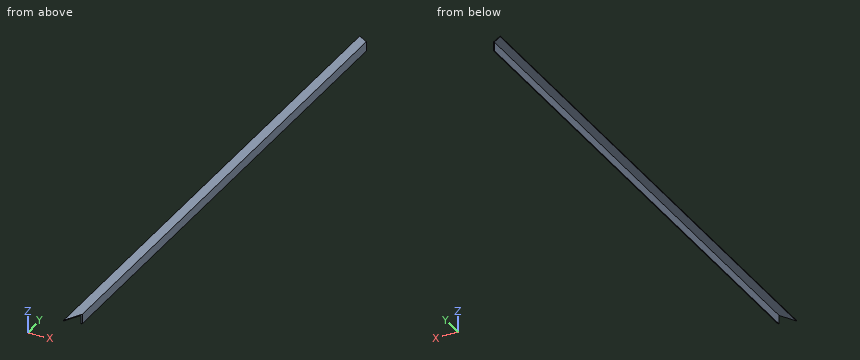
Autodesk Inventor part; units mm, degrees
ref_plane "YZ Plane" through (0, 0, 0) normal (1, 0, 0) x (0, 1, 0)
ref_plane "XZ Plane" through (0, 0, 0) normal (0, 1, 0) x (-1, 0, 0)
ref_plane "XY Plane" through (0, 0, 0) normal (0, 0, 1) x (1, 0, 0)
sketch "Sketch1" plane through (0, 0, 0) normal (0, 1, 0) x (-1, 0, 0)
  line L0 (0, 0) -> (38.1, 0)
  line L1 (38.1, 0) -> (38.1, -3.175)
  line L2 (38.1, -3.175) -> (3.175, -3.175)
  line L3 (3.175, -3.175) -> (3.175, -38.1)
  line L4 (3.175, -38.1) -> (0, -38.1)
  line L5 (0, -38.1) -> (0, 0)
  dimension "d0" = 3.175
  dimension "d1" = 3.175
  dimension "d2" = 38.1
  dimension "d3" = 38.1
extrude "Extrusion1" add sketch "Sketch1" along normal blind 2133.6
sketch "Sketch2" plane through (0, 0, 0) normal (0, 0, 1) x (1, 0, 0)
  line L0 (0, 0) -> (-38.1, 0)
  line L1 (-38.1, 0) -> (0, 0)
  line L2 (0, 0) -> (-38.1, 0)
  line L3 (-38.1, 0) -> (0, 65.9911)
  line L4 (0, 0) -> (0, 2133.6)
  line L5 (-38.1, 0) -> (-38.1, 2133.6)
  line L6 (-38.1, 2133.6) -> (0, 2111.603)
  line L7 (-38.1, 2133.6) -> (0, 2133.6)
  line L8 (0, 2111.603) -> (0, 2133.6)
  line L9 (0, 2133.6) -> (-38.1, 2133.6)
  dimension "d6" = 60
  dimension "d7" = 60
extrude "Extrusion2" cut sketch "Sketch2" against normal blind 76.2 contours L0 L3 L4
extrude "Extrusion3" cut sketch "Sketch2" against normal blind 76.2 contours L7 L4 L6
properties part number "Angle_Brace"
Input: part model. Units: mm. Frame: model coordinates. Coordinates: 2 decimals unless noted, no trailing zeros. Loops run counter-clockwise (first coordinate to the right, second up) from the corner with the lowest first, then second, coordinate; pieces in that order, holes last. Notation, with made-up numbers: (64, 71) - (74, 71) arc R20 cw to (74, 91) - close; hole circle Ø8 at (39.25, 24). An arc over 180 degrees is marked (long way). Answer in a Markdown table with one row per item. Add a question column.
Item 1: Line query: line 1 along X through (y, z) = (1760, -18) (3 decimals); line 2 along Y through (x, z) = (-5.5, -2). Output: solid intervals per line, ascending. Write a range as [from, to].
Item 2: Section query B-B on z = -12.5. Return the cut outline in (x, y) (3 decimals), then the cut area to 3 significant figures.
Item 3: Section query C-C on x = -20.5. Return the cut outline in (y, z) (3 decimals), then the cut area to 3 significant figures.
Item 4: Section query A-A on y = 509.5. Return the cut outline in (x, z) (3 decimals), then the cut area to 3 significant figures.
Item 5: Contact query for flat-ended pins moving along their axis: P1, Ø12, axis at y = 1236, z = -12, coming from the +X side; P2, Ø4, axis at x = -13, z = -5, coming from the +Y side; P3, Ø6, axis at y = 1079.5, z = -14.5, coming from the -X side (3 decimals). Output: stop coordinate, or through.
Recorded:
| question | item | result |
|---|---|---|
| 1 | line 1 | [-3.175, 0] |
| 1 | line 2 | [56.46, 2114.78] |
| 2 | outline | (-3.175, 60.492) - (0, 65.991) - (0, 2111.603) - (-3.175, 2113.436) - close |
| 2 | area | 6,510 mm^2 |
| 3 | outline | (30.484, -3.175) - (2123.439, -3.175) - (2123.439, 0) - (30.484, 0) - close |
| 3 | area | 6,650 mm^2 |
| 4 | outline | (-38.1, -3.175) - (-3.175, -3.175) - (-3.175, -38.1) - (0, -38.1) - (0, 0) - (-38.1, 0) - close |
| 4 | area | 232 mm^2 |
| 5 | P1 | x = 0 |
| 5 | P2 | y = 2119.58 |
| 5 | P3 | x = -3.175 |
